Design review of the part built by this model. Coordinates are the model's own, in mm. A direction names the side the tool comes from. Round coordinates to 2 decimals unless told otherwise and drop trailing zeros. Order: outer loops, then holes, each group sorted by start corner. A loop starts at its lowest first (then second) coordinate and runs counter-clockwise, first axis right, second up.
from build123d import *

# Parameters (mm, degrees)
F1_DEPTH  = 0.762
F2_R      = 1.905
F4_DEPTH  = 19.05
F5_R      = 1.905
F7_DEPTH  = 25.4
F8_R      = 1.905
F12_DEPTH = 25.4
F11_R     = 3.175
F11_R_2   = 1.27
F13_DEPTH = 5.334


with BuildPart() as f1:
    # F0 (on Top) → F1 (new body)
    with BuildSketch(Plane.XY):
        Polygon((19.05, 32.995568), (-19.05, 32.995568), (-38.1, 0), (-19.05, -32.995568), (19.05, -32.995568), (38.1, 0), align=None)
    extrude(amount=F1_DEPTH)

    # F2
    f2_edges = [f1.edges().sort_by_distance(p)[0] for p in [
        (38.1, 0, 0.381),
        (19.05, 32.995568, 0.381),
        (-19.05, 32.995568, 0.381),
        (-38.1, 0, 0.381),
        (-19.05, -32.995568, 0.381),
        (19.05, -32.995568, 0.381),
    ]]
    fillet(f2_edges, radius=F2_R)


with BuildPart() as f4:
    # F3 (on Top) → F4 (new body)
    with BuildSketch(Plane.XY):
        Polygon((18.415, 31.895716), (-18.415, 31.895716), (-36.83, 0), (-18.415, -31.895716), (18.415, -31.895716), (36.83, 0), align=None)
    extrude(amount=F4_DEPTH)

    # F5
    f5_edges = [f4.edges().sort_by_distance(p)[0] for p in [
        (-18.415, -31.895716, 9.525),
        (18.415, -31.895716, 9.525),
        (36.83, 0, 9.525),
        (-36.83, 0, 9.525),
        (18.415, 31.895716, 9.525),
        (-18.415, 31.895716, 9.525),
    ]]
    fillet(f5_edges, radius=F5_R)


with BuildPart() as f7:
    # F6 (on Top) → F7 (new body)
    with BuildSketch(Plane.XY):
        Polygon((17.907, 31.015834), (-17.907, 31.015834), (-35.814, 0), (-17.907, -31.015834), (17.907, -31.015834), (35.814, 0), align=None)
    extrude(amount=F7_DEPTH)

    # F8
    f8_edges = [f7.edges().sort_by_distance(p)[0] for p in [
        (-17.907, -31.015834, 12.7),
        (17.907, -31.015834, 12.7),
        (35.814, 0, 12.7),
        (-35.814, 0, 12.7),
        (17.907, 31.015834, 12.7),
        (-17.907, 31.015834, 12.7),
    ]]
    fillet(f8_edges, radius=F8_R)


with BuildPart() as f7_1:
    # F9: moved
    add(f7.part.moved(Location((0, 0, 0.762))))


with BuildPart() as f4_1:
    add(f4.part)

    # F10: cut F7
    add(f7_1.part, mode=Mode.SUBTRACT)


with BuildPart() as f12_tool:
    # F11 (on face) → F12 (new body)
    with BuildSketch(Plane.XY.offset(0.762)):
        Polygon((-1.175437, 0), (1.175437, 0), (2.350874, 2.035916), (1.175437, 4.071832), (-1.175437, 4.071832), (-2.350874, 2.035916), align=None)
    extrude(amount=-F12_DEPTH)


with BuildPart() as f1_1:
    add(f1.part)

    # F12: cut by f12_tool
    add(f12_tool.part, mode=Mode.SUBTRACT)



with BuildPart() as f4_2:
    add(f4_1.part)

    # F12: cut by f12_tool
    add(f12_tool.part, mode=Mode.SUBTRACT)


with BuildPart() as f1_2:
    add(f1_1.part)

    add(f4_2.part)  # F13 merges F4
    # F11 (on face) → F13 (join)
    with BuildSketch(Plane.XY.offset(0.762)):
        with Locations((-9.2075, 4.163166)):
            Circle(F11_R)
        with Locations((-9.2075, 4.163166)):
            Circle(F11_R_2, mode=Mode.SUBTRACT)
        with Locations((9.2075, 4.163166)):
            Circle(F11_R)
        with Locations((9.2075, 4.163166)):
            Circle(F11_R_2, mode=Mode.SUBTRACT)
        with Locations((9.2075, -27.586834)):
            Circle(F11_R)
        with Locations((9.2075, -27.586834)):
            Circle(F11_R_2, mode=Mode.SUBTRACT)
        with Locations((-9.2075, -27.586834)):
            Circle(F11_R)
        with Locations((-9.2075, -27.586834)):
            Circle(F11_R_2, mode=Mode.SUBTRACT)
    extrude(amount=F13_DEPTH)


solid = f1_2.part
1) To check wall thickness, follow line 1 along Y through (x, z) = (1.5, 5.5); line 2 along Z through (x, y) = (-25, 10.5); line 3 along Y through (x, z) = (23.5, 11.75). State the ranges of each line that lie inside material, in increasing order.
Results:
line 1: y = -31.9 to -31.02, 31.02 to 31.9
line 2: z = 0 to 0.76
line 3: y = -23.09 to -21.33, 21.33 to 23.09
2) For faces 1 (the face through (27.5, -16.16, 9.78)), 2 (the face through (8.932, -28.827, 3.392)), 3 (the face through (-28.449, 16.715, 0.376)), 4 (the face through (-27.744, -15.738, 9.778)), list the 3-axis set-ups (+Z, -Z, +X, -X, +Y, -Y) from which the entire face can be reached by the end or side of a thin tool; tool diameter is ignored.
Results:
face 1: +Z, +X, -Y
face 2: +Z
face 3: +Z, -Z, -X, +Y
face 4: +Z, -X, -Y
3) The part is to be moulded in two halves that separate along X. For faces 5 (the face through (27, -16, 19.05)), 6 (the face through (26.98, 15.3, 9.78)), 7 (the face through (-28.7, -16.28, 0.38)), say which applies: released by +X, released by -X, zero draft, split by the parting line, or undercut.
Results:
face 5: zero draft
face 6: undercut
face 7: released by -X
4) Take a section at C-C on z = 10.25. Give the boundary of the cut face in (x, y) (1 decimal).
Results:
outline: (-36.3, -1) - (-19, -30.9) arc R1.9 ccw to (-17.3, -31.9) - (17.3, -31.9) arc R1.9 ccw to (19, -30.9) - (36.3, -1) arc R1.9 ccw to (36.3, 1) - (19, 30.9) arc R1.9 ccw to (17.3, 31.9) - (-17.3, 31.9) arc R1.9 ccw to (-19, 30.9) - (-36.3, 1) arc R1.9 ccw to start; hole (-35.3, -1) - (-18.5, -30.1) arc R1.9 ccw to (-16.8, -31) - (16.8, -31) arc R1.9 ccw to (18.5, -30.1) - (35.3, -1) arc R1.9 ccw to (35.3, 1) - (18.5, 30.1) arc R1.9 ccw to (16.8, 31) - (-16.8, 31) arc R1.9 ccw to (-18.5, 30.1) - (-35.3, 1) arc R1.9 ccw to start
5) Take a section at A-A on z = 5.25. State how many separate pieces and enclosed holes the cut face has, plus the area to 3 significant figures.
Results:
separate pieces: 5
enclosed holes: 5
area: 298 mm2
6) Clearance check with flat-ended pins moving along their axes: P1, Ø1.3, axis at x = 9, y = -28, coming from the +Z side; P2, Ø5, axis at x = -10, y = -27, coming from the +Z side; P3, Ø9, axis at x = 3.5, z = 11.5, coming from the -Y side. State where each tip first meets the part, or that it passes through.
Results:
P1: stops at z = 0.76
P2: stops at z = 6.1
P3: stops at y = -31.9
7) Take a section at B-B on x = -13.5. Give the boundary of the cut face in (y, z), plus the area to 3 significant figures.
Results:
outline: (-33, 0) - (33, 0) - (33, 0.76) - (31.9, 0.76) - (31.9, 19.05) - (31.02, 19.05) - (31.02, 0.76) - (-31.02, 0.76) - (-31.02, 19.05) - (-31.9, 19.05) - (-31.9, 0.76) - (-33, 0.76) - close
area: 82.5 mm2
8) Take a section at D-D on y = -14.5. Give the boundary of the cut face in (x, z).
Results:
outline: (-29.73, 0) - (29.73, 0) - (29.73, 0.76) - (28.46, 0.76) - (28.46, 19.05) - (27.44, 19.05) - (27.44, 0.76) - (-27.44, 0.76) - (-27.44, 19.05) - (-28.46, 19.05) - (-28.46, 0.76) - (-29.73, 0.76) - close
